Model file for the job. Use its own axes, mm. Face numbers are marked on the shaded views. A direction names the side the tool comes from. Round coordinates to 2 decimals unless told otherwise and drop trailing zeros. Order: outer loops, then holes, each group sorted by start corner. A loop starts at its lowest first (then second) coordinate and runs counter-clockwise, first axis right, second up. Notation, with made-up numbers: (42.25, -38.5) -> (99.25, -38.5) arc R28 cw to (99.25, -19.5) -> close; hole circle Ø7 at (50.25, -17.75). An arc over 180 degrees is marked (long way). Put each result on its own line as item: value. Start each with the question number.
Q1. Cut at D-D, the plane z = -27. List the corners of the cut face in (x, y).
Q2. Cut at B-B, the plane x = -13.76. List the corners of the cut face in (y, z).
Q3. Cut at C-C, the plane y = -4.5. List the corners of the cut face in (x, z).
Q4. Probe L1, parallel to X at y = 12, z = 0; L2, parallel to Z at x = -13.76, y = 5; L3, parallel to X at y = 6.5, z = 0. List the from-to ranges inside material, lowest first.
Q5. 3-axis set-ups, long thin cutter, end or side, ignore diameter. For the marked faces 1, 2 and 3: which of +Z, -Z, +X, -X, +Y, -Y reach the whole face in a straight line?
Q6. Cut at A-A, the plane z = 0. List the corners of the cut face in (x, y).
Q7. Pull direction Z, two halves, no side cores. Call the marked faces 4, 5 and 6: released by +Z, released by -Z, zero draft, split by the parting line, or undercut.
Q8. Flat gauge pins, fed straight in: P1, Ø14.5, axis at x = 13.76, z = 0, coming from the -Y side; P2, Ø1.5, axis at y = 11.5, z = 19.5, coming from the -X side; P3, Ø3, axis at x = 58, z = 32.5, coming from the -Y side; P4, Ø4, axis at y = 12.5, z = 17.5, coming from the +X side. Where does each tip first touch, or does it go through?
from build123d import *

# Parameters (mm, degrees)
SKETCH1_W               = 210
SKETCH1_H               = 100
BOSS_EXTRUDE1_DEPTH     = 10
SKETCH2_W               = 190
SKETCH2_H               = 80
BOSS_EXTRUDE2_DEPTH     = 5
SKETCH3_W               = 57
SKETCH3_H               = 32
SKETCH3_W_2             = 47
SKETCH3_H_2             = 22
BOSS_EXTRUDE3_DEPTH     = 15
CUT_EXTRUDE1_DEPTH      = 118.260393996
CUT_EXTRUDE1_DEPTH_BACK = 118.260393996
SKETCH4_R               = 8


with BuildPart() as part:
    # Sketch1 → Boss-Extrude1 (new body)
    with BuildSketch(Plane(origin=(0, 0, 0), x_dir=(1, 0, 0), z_dir=(0, 1, 0))):
        Rectangle(SKETCH1_W, SKETCH1_H)
    extrude(amount=BOSS_EXTRUDE1_DEPTH)

    # Sketch2 → Boss-Extrude2 (add)
    with BuildSketch(Plane(origin=(0, 10, 0), x_dir=(1, 0, 0), z_dir=(0, 1, 0))):
        Rectangle(SKETCH2_W, SKETCH2_H)
    extrude(amount=BOSS_EXTRUDE2_DEPTH)

    # Sketch3 → Boss-Extrude3 (add)
    with BuildSketch(Plane.XZ):
        Rectangle(SKETCH3_W, SKETCH3_H)
        Rectangle(SKETCH3_W_2, SKETCH3_H_2, mode=Mode.SUBTRACT)
    extrude(amount=BOSS_EXTRUDE3_DEPTH)

    # Sketch4 → Cut-Extrude1 (cut, two sides: drawn at the far end of the back side and taken through both)
    with BuildSketch(Plane.XZ.offset(-CUT_EXTRUDE1_DEPTH_BACK)):
        with Locations(Location((-13.76, 0, 0), (0, 0, 270))):
            Circle(SKETCH4_R)
        with Locations(Location((13.76, 0, 0), (0, 0, 90))):
            Circle(SKETCH4_R)
    extrude(amount=CUT_EXTRUDE1_DEPTH + CUT_EXTRUDE1_DEPTH_BACK, mode=Mode.SUBTRACT)


solid = part.part
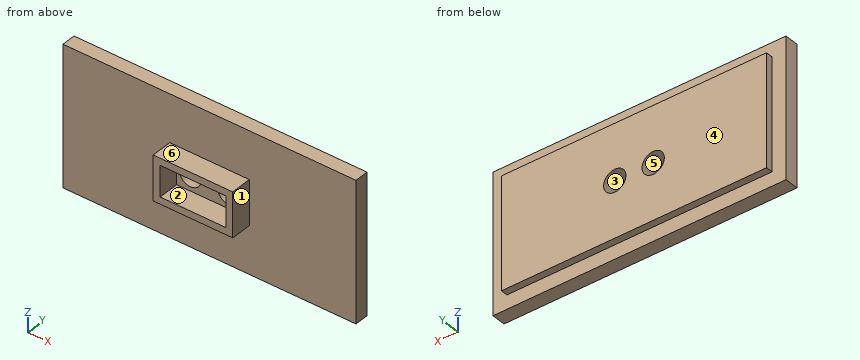
Ans:
1. outline: (-105, 0) -> (105, 0) -> (105, 10) -> (95, 10) -> (95, 15) -> (-95, 15) -> (-95, 10) -> (-105, 10) -> close
2. outline: (-15, -16) -> (0, -16) -> (0, -50) -> (10, -50) -> (10, -40) -> (15, -40) -> (15, -8) -> (0, -8) -> (0, -11) -> (-15, -11) -> close; (-15, 11) -> (0, 11) -> (0, 8) -> (15, 8) -> (15, 40) -> (10, 40) -> (10, 50) -> (0, 50) -> (0, 16) -> (-15, 16) -> close
3. outline: (-28.5, -16) -> (28.5, -16) -> (28.5, 16) -> (-28.5, 16) -> close; hole (-23.5, -11) -> (23.5, -11) -> (23.5, 11) -> (-23.5, 11) -> close
4. L1: x = -95 to -21.76, -5.76 to 5.76, 21.76 to 95
4. L2: z = -50 to -8, 8 to 50
4. L3: x = -105 to -21.76, -5.76 to 5.76, 21.76 to 105
5. face 1: +Z, -Z, +X, -Y
5. face 2: -Y
5. face 3: +Y, -Y
6. outline: (-105, 0) -> (-28.5, 0) -> (-28.5, -15) -> (-23.5, -15) -> (-23.5, 0) -> (-21.76, 0) -> (-21.76, 15) -> (-95, 15) -> (-95, 10) -> (-105, 10) -> close; (-5.76, 0) -> (5.76, 0) -> (5.76, 15) -> (-5.76, 15) -> close; (21.76, 0) -> (23.5, 0) -> (23.5, -15) -> (28.5, -15) -> (28.5, 0) -> (105, 0) -> (105, 10) -> (95, 10) -> (95, 15) -> (21.76, 15) -> close
7. face 4: zero draft
7. face 5: undercut
7. face 6: released by +Z
8. P1: passes through
8. P2: stops at x = -95
8. P3: stops at y = 0
8. P4: stops at x = 95
